```python
from build123d import *

# Parameters (mm, degrees)
EXTRU_MINCE1_DEPTH      = 25
EXTRU_MINCE1_DEPTH_BACK = 25


with BuildPart() as part:
    # Esquisse2 → Extru.-Mince1 (new body, two sides)
    with BuildSketch(Plane.XY) as extru_mince1_sk:
        with BuildLine():
            Line((-272.299999984, 13.855), (272.300004367, 13.855))
            ThreePointArc((272.300004367, 13.855), (286.155004367, -2.192e-06), (272.299999984, -13.855))
            Line((272.299999984, -13.855), (-272.300004367, -13.855))
            ThreePointArc((-272.300004367, -13.855), (-286.155004367, 2.192e-06), (-272.299999984, 13.855))
        make_face()
        with BuildLine():
            Line((-272.3, 13.755), (272.3, 13.755))
            ThreePointArc((272.3, 13.755), (286.055004367, 0), (272.3, -13.755))
            Line((272.3, -13.755), (-272.3, -13.755))
            ThreePointArc((-272.3, -13.755), (-286.055004367, 0), (-272.3, 13.755))
        make_face(mode=Mode.SUBTRACT)
    extrude(amount=EXTRU_MINCE1_DEPTH)
    extrude(extru_mince1_sk.sketch, amount=-EXTRU_MINCE1_DEPTH_BACK)


solid = part.part
```
Geometry check sheet. Reference: the model listing, model coordinates, mm. Coordinates: 2 decimals unless noted, no trailing zeros. Order: outer loops, then holes, each group sorted by start corner. A loop starts at its lowest first (then second) coordinate and runs counter-clockwise, first axis right, second up. Notation, with made-up numbers: (-2.5, -9.5) - (5.5, -9.5) arc R15 cw to (5.5, 7.5) - close; hole circle Ø5 at (12, 57). An arc over 180 degrees is marked (long way). Answer as a JSON object with one key per item and string values. Group by question number.
Item 1: Sectioned sample at C-C, the plane z = 11. Record the cut outline in (x, y) (3 decimals).
Item 2: Sectioned sample at B-B, the plane y = 0. Record the cut outline in (x, z) (3 decimals).
Item 3: Sectioned sample at A-A, the plane x = -232.5. Record the cut outline in (y, z) (3 decimals), and give its area (3 significant figures).
Item 4: Scan lines: probe 1 along X at (y, z) = (-11, 8.5); probe 2 along X at (y, z) = (11.25, 3). Record each from-to range of solid material in increasing order.
Resolved:
{
 "1": {"outline": "(-272.3, -13.855) - (272.3, -13.855) arc R13.855 ccw to (272.3, 13.855) - (-272.3, 13.855) arc R13.855 ccw to start; hole (-272.3, -13.755) - (272.3, -13.755) arc R13.755 ccw to (272.3, 13.755) - (-272.3, 13.755) arc R13.755 ccw to start"},
 "2": {"outline": "(-286.155, -25) - (-286.055, -25) - (-286.055, 25) - (-286.155, 25) - close; (286.055, -25) - (286.155, -25) - (286.155, 25) - (286.055, 25) - close"},
 "3": {"outline": "(-13.855, -25) - (-13.755, -25) - (-13.755, 25) - (-13.855, 25) - close; (13.755, -25) - (13.855, -25) - (13.855, 25) - (13.755, 25) - close", "area": "10.0 mm^2"},
 "4": {"probe 1": "-280.72 to -280.56, 280.56 to 280.72", "probe 2": "-280.39 to -280.21, 280.21 to 280.39"}
}
